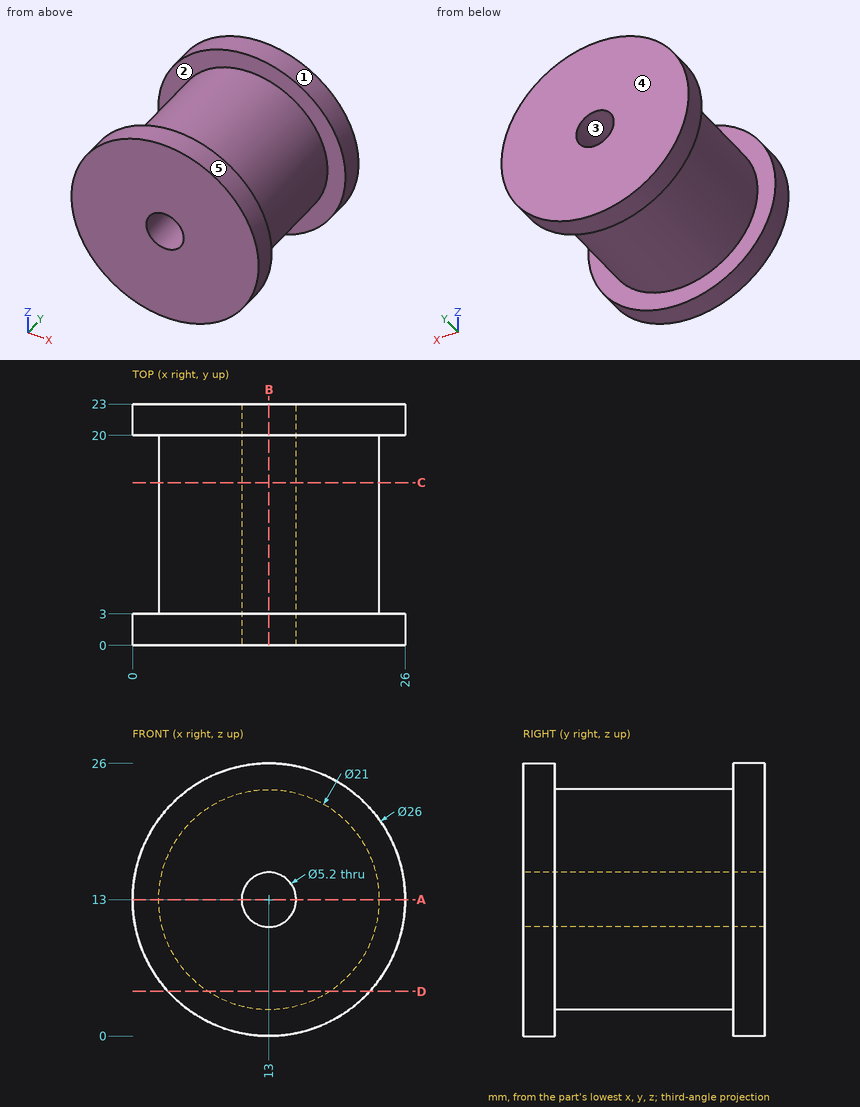
Part print with two shaded views. Sizes in mm from the minimum x, y, z corner. A direction names the side the tool comes from. Coordinates: 2 decimals unless noted, no trailing zeros. Write each loop counter-clockwise with the first axis right and the second up, starting at its lowest first coordinate (ties: lowest second). Pieces come first, ordered by that corner, then holes.
1. 3-axis set-ups, long thin cutter, end or side, ignore diameter. For the marked faces 1 and 2: which of +Z, -Z, +X, -X, +Y, -Y reach the whole face in a straight line?
Answer block:
face 1: +Y, -Y
face 2: none
2. Pull direction Z, two halves, no side cores. Call the marked faces 3, 4 and 5: released by +Z, released by -Z, zero draft, split by the parting line, or undercut.
Answer block:
face 3: undercut
face 4: zero draft
face 5: split by the parting line
3. Band-saw the part on A-A, the plane z = 13. Give the cut face in (x, y).
Answer block:
outline: (0, 0) - (10.4, 0) - (10.4, 23) - (0, 23) - (0, 20) - (2.5, 20) - (2.5, 3) - (0, 3) - close; (15.6, 0) - (26, 0) - (26, 3) - (23.5, 3) - (23.5, 20) - (26, 20) - (26, 23) - (15.6, 23) - close
4. Band-saw the part on D-D, the plane z = 4.25. Give the cut face in (x, y).
Answer block:
outline: (3.39, 0) - (22.61, 0) - (22.61, 3) - (18.8, 3) - (18.8, 20) - (22.61, 20) - (22.61, 23) - (3.39, 23) - (3.39, 20) - (7.2, 20) - (7.2, 3) - (3.39, 3) - close
5. Drop flat-ended pins along their axis: pin 1 (1 mm diameter, centred on x = 21, y = 14.5, fed in from +Z); pin 2 (6 mm diameter, centred on y = 5, z = 15.5, fed in from -X); pin 3 (5 mm diameter, centred on x = 11.5, y = 17, fed in from +Z); pin 4 (4 mm diameter, centred on x = 13, z = 13, fed in from +Y). Give the stop position or say it passes through.
Answer block:
pin 1: stops at z = 20.35
pin 2: stops at x = 0
pin 3: stops at z = 23.5
pin 4: passes through
6. Band-saw the part on B-B, the plane x = 13. Give the cut face in (y, z).
Answer block:
outline: (0, 0) - (3, 0) - (3, 2.5) - (20, 2.5) - (20, 0) - (23, 0) - (23, 10.4) - (0, 10.4) - close; (0, 15.6) - (23, 15.6) - (23, 26) - (20, 26) - (20, 23.5) - (3, 23.5) - (3, 26) - (0, 26) - close
7. Band-saw the part on C-C, the plane y = 15.5. Give the cut face in (x, z), and give its area (3 significant figures).
Answer block:
outline: circle Ø21 at (13, 13); hole circle Ø5.2 at (13, 13)
area: 325 mm2
8. Drill centre lines: probe 1 along Z at (x, y) = (13, 15); probe 2 along Y at (x, z) = (24, 15.5); probe 3 along Z at (x, y) = (12.25, 10). Where is each one in solid material? Low to high.
Answer block:
probe 1: z = 2.5 to 10.4, 15.6 to 23.5
probe 2: y = 0 to 3, 20 to 23
probe 3: z = 2.53 to 10.51, 15.49 to 23.47
